```python
from build123d import *

# Parameters (mm, degrees)
SKETCH1_W                              = 25
SKETCH1_H                              = 75
BOSS_EXTRUDE1_DEPTH                    = 4
SKETCH2_W                              = 5
SKETCH2_H                              = 20.2
CUT_EXTRUDE1_DEPTH                     = 41.32988966
SKETCH3_W                              = 25
SKETCH3_H                              = 9
CUT_EXTRUDE2_DEPTH                     = 4.8
FILLET1_R                              = 2.5
CHAMFER1_SIZE                          = 2
TAPPED_HOLE_FOR_M4X0_7_HELICOIL1_D     = 4.2
TAPPED_HOLE_FOR_M4X0_7_HELICOIL1_DEPTH = 6.8
TAPPED_HOLE_FOR_M4X0_7_HELICOIL1_TIP   = 1.2618073
M4_CLEARANCE_HOLE1_D                   = 4.2


with BuildPart() as part:
    # Sketch1 → Boss-Extrude1 (new, symmetric)
    with BuildSketch(Plane.XY):
        Rectangle(SKETCH1_W, SKETCH1_H)
    extrude(amount=BOSS_EXTRUDE1_DEPTH, both=True)

    # Sketch2 → Cut-Extrude1 (cut, through all)
    with BuildSketch(Plane.XY.offset(4)):
        with Locations((-10, 27.4)):
            Rectangle(SKETCH2_W, SKETCH2_H)
    extrude(amount=-CUT_EXTRUDE1_DEPTH, mode=Mode.SUBTRACT)

    # Sketch3 → Cut-Extrude2 (cut)
    with BuildSketch(Plane.XY.offset(4)):
        with Locations((0, -33)):
            Rectangle(SKETCH3_W, SKETCH3_H)
    extrude(amount=-CUT_EXTRUDE2_DEPTH, mode=Mode.SUBTRACT)

    # Fillet1
    fillet1_edges = [part.edges().sort_by_distance(p)[0] for p in [
        (12.5, 37.5, 0),
    ]]
    fillet(fillet1_edges, radius=FILLET1_R)

    # Chamfer1
    chamfer1_edges = [part.edges().sort_by_distance(p)[0] for p in [
        (12.5, -37.5, -2.4),
        (-12.5, -37.5, -2.4),
    ]]
    chamfer(chamfer1_edges, length=CHAMFER1_SIZE)

    # Tapped Hole for M4x0.7 Helicoil1
    with Locations(Plane.ZY.offset(7.5)):
        with Locations((0, 22.5), (0, 32.5)):
            Hole(TAPPED_HOLE_FOR_M4X0_7_HELICOIL1_D / 2, depth=TAPPED_HOLE_FOR_M4X0_7_HELICOIL1_DEPTH)
            with Locations((0, 0, -(TAPPED_HOLE_FOR_M4X0_7_HELICOIL1_DEPTH + TAPPED_HOLE_FOR_M4X0_7_HELICOIL1_TIP / 2))):  # 118° drill point
                Cone(0, TAPPED_HOLE_FOR_M4X0_7_HELICOIL1_D / 2, TAPPED_HOLE_FOR_M4X0_7_HELICOIL1_TIP, mode=Mode.SUBTRACT)

    # M4 Clearance Hole1 (through all)
    with Locations(Plane(origin=(0, 0, -4), x_dir=(-1, 0, 0), z_dir=(0, 0, -1))):
        with Locations((-6.483, -32.5028), (3.517, -32.5028)):
            Hole(M4_CLEARANCE_HOLE1_D / 2)


solid = part.part
```
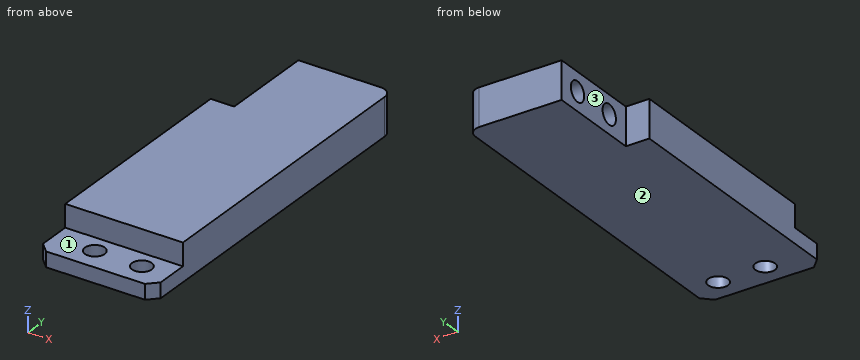
Geometry check sheet. Reference: the model listing, model coordinates, mm. Face numbers are marked on the shaded views. A direction names the side the tool comes from. Give positions to 0.01 mm unless a question says otherwise; leave off trailing zeros. Write each loop counter-clockwise with the first axis right and the second up, starting at its lowest first coordinate (ties: lowest second). Pieces come first, ordered by that corner, then holes.
1) Material ranges on L1, parallel to Y at x = -2, z = -0.25; L2, parallel to Z at x = -2, y = 22.5; L3, parallel to Y at x = 9.25, z = 2.5, recorded low to high.
2) Access from +Z, -Z, +X, -X, +Y, -Y to the whole of each face (thin tool, end or side, straight path). Record for the marked faces 1, 2 and 3.
3) Section check B-B, the plane x = 5.5. Record the boundary of the cut face in (y, z), and give its area (3 significant figures).
4) Gauge pin test, flat ends, axial feed: pin 1 (2.5 mm diameter, centred on x = 5, y = -33.5, fed in from +Z); pin 2 (5.5 mm diameter, centred on x = 6.48, y = -32.5, fed in from -Z); pin 3 (4 mm diameter, centred on y = 27, z = 2, fed in from -X); pin 4 (4 mm diameter, centred on x = -10, z = 2, fed in from +Y). Record the tip position at first contact, or that the pin passes through.
5) Section check A-A, the plane x = -6.75. Record the boundary of the cut face in (y, z).
6) Section check D-D, the plane y = -29.5. Record the boundary of the cut face in (x, z).
7) Section check C-C, the plane y = 18. Record the boundary of the cut face in (x, z).
Computed:
1. L1: y = -28.5 to 20.41, 24.59 to 30.41, 34.59 to 37.5
1. L2: z = -4 to -2.1, 2.1 to 4
1. L3: y = -28.5 to 37.5
2. face 1: +Z, +X, -X, -Y
2. face 2: -Z, +X, -X, +Y, -Y
2. face 3: +Z, -Z, -X, +Y
3. outline: (-37.5, -4) - (-34.36, -4) - (-34.36, -0.8) - (-37.5, -0.8) - close; (-30.65, -4) - (37.5, -4) - (37.5, 4) - (-28.5, 4) - (-28.5, -0.8) - (-30.65, -0.8) - close
3. area: 545 mm2
4. pin 1: stops at z = -0.8
4. pin 2: stops at z = -4
4. pin 3: stops at x = -7.5
4. pin 4: stops at y = 17.3
5. outline: (-37.5, -4) - (37.5, -4) - (37.5, 4) - (-28.5, 4) - (-28.5, -0.8) - (-37.5, -0.8) - close; hole circle Ø4.2 at (22.5, 0); hole circle Ø4.2 at (32.5, 0)
6. outline: (-12.5, -4) - (12.5, -4) - (12.5, -0.8) - (-12.5, -0.8) - close
7. outline: (-7.5, -4) - (12.5, -4) - (12.5, 4) - (-7.5, 4) - close
